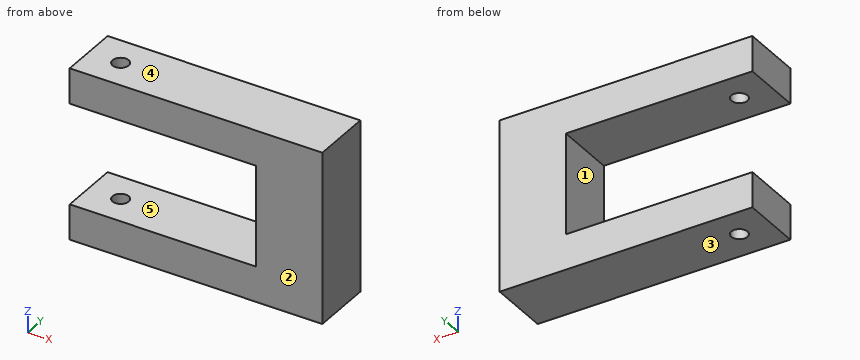
from build123d import *

# Parameters (mm, degrees)
EXTRUDE_START       = 7.5
SKETCH_1_W          = 125.131658012
SKETCH_1_H          = 30
EXTRUDE_1_DEPTH     = 85
SKETCH_3_W          = 94.594294475
SKETCH_3_H          = 50
CUT_EXTRUDE_1_DEPTH = 43.5
SKETCH_4_R          = 4
CUT_EXTRUDE_2_DEPTH = 100


with BuildPart() as part:
    # Эскиз1 → Вытянуть1 (new body)
    with BuildSketch(Plane.XY.offset(EXTRUDE_START)):
        with Locations((62.565829006, -9.041900761)):
            Rectangle(SKETCH_1_W, SKETCH_1_H)
    extrude(amount=-EXTRUDE_1_DEPTH)

    # Эскиз3 → Вырез-Вытянуть1 (cut, symmetric)
    with BuildSketch(Plane(origin=(0, 0, 0), x_dir=(1, 0, 0), z_dir=(0, 1, 0))):
        with Locations((45.031047777, 35)):
            Rectangle(SKETCH_3_W, SKETCH_3_H)
    extrude(amount=CUT_EXTRUDE_1_DEPTH, both=True, mode=Mode.SUBTRACT)

    # Эскиз4 → Вырез-Вытянуть2 (cut, symmetric)
    with BuildSketch(Plane.XY):
        with Locations((15.823953055, -9.041900761)):
            Circle(SKETCH_4_R)
    extrude(amount=CUT_EXTRUDE_2_DEPTH, both=True, mode=Mode.SUBTRACT)


solid = part.part
CAD build for the part. Positions are in the model's coordinates, mm. Face numbers are marked on the shaded views. A direction names the side the tool comes from. Give positions to 0.01 mm unless a question says otherwise; leave off trailing zeros. Write each loop counter-clockwise with the first axis right and the second up, starting at its lowest first coordinate (ties: lowest second). Pieces come first, ordered by that corner, then holes. Notation, with made-up numbers: (6, 16) - (43, 16) arc R20 cw to (43, 26) - close; hole circle Ø11 at (55.5, 86). An arc over 180 degrees is marked (long way). Put each result on its own line as item: value.
(1) Saw through at B-B (y = -17). List the corners of the cut face in (x, z), then the cut area to 3 significant figures.
Working result:
outline: (0, -77.5) - (125.13, -77.5) - (125.13, 7.5) - (0, 7.5) - (0, -10) - (92.33, -10) - (92.33, -60) - (0, -60) - close
area: 6,020 mm^2
(2) Pull direction Z, two halves, no side cores. Call the marked faces 1, 2 and 3: released by +Z, released by -Z, zero draft, split by the parting line, or undercut.
Working result:
face 1: undercut
face 2: zero draft
face 3: released by -Z
(3) Tool access for the marked faces 4 and 5: list every direction of +Z, -Z, +X, -X, +Y, -Y with a clear straight run to the whole face (end or side of a thin tool).
Working result:
face 4: +Z, +X, -X, +Y, -Y
face 5: -X, +Y, -Y
(4) Saw through at C-C (y = -7.25). List the corners of the cut face in (x, z).
Working result:
outline: (0, -77.5) - (12.25, -77.5) - (12.25, -60) - (0, -60) - close; (0, -10) - (12.25, -10) - (12.25, 7.5) - (0, 7.5) - close; (19.4, -77.5) - (125.13, -77.5) - (125.13, 7.5) - (19.4, 7.5) - (19.4, -10) - (92.33, -10) - (92.33, -60) - (19.4, -60) - close
(5) Saw through at D-D (z = -53). List the corners of the cut face in (x, y).
Working result:
outline: (92.33, -24.04) - (125.13, -24.04) - (125.13, 5.96) - (92.33, 5.96) - close
(6) Drop flat-ended pins along their axis: pin 1 Ø12 at (y, z) = (2.5, -40.5) entering from -X; pin 2 Ø12 at (y, z) = (3, -2.5) entering from -X. Give the stop position or say it passes through.
Working result:
pin 1: x = 92.33
pin 2: x = 0
(7) Wall check: L1, parallel to Z at x = 80, y = -2.75; L2, parallel to X at y = 1, z = -57.5; L3, parallel to X at y = -9.5, z = 4.5. Give the ranges that are in metal, low to high.
Working result:
L1: -77.5 to -60, -10 to 7.5
L2: 92.33 to 125.13
L3: 0 to 11.85, 19.8 to 125.13
(8) Saw through at A-A (x = 29). List the corners of the cut face in (y, z).
Working result:
outline: (-24.04, -77.5) - (5.96, -77.5) - (5.96, -60) - (-24.04, -60) - close; (-24.04, -10) - (5.96, -10) - (5.96, 7.5) - (-24.04, 7.5) - close
